Build history of the part. All positions in model axes, mm. A direction names the side the tool comes from. Round coordinates to 2 decimals unless told otherwise and drop trailing zeros. Write each loop counter-clockwise with the first axis right and the second up, starting at its lowest first coordinate (ties: lowest second). Pieces come first, ordered by that corner, then holes.
1) Which spindle directions (+Z, -Z, +X, -X, +Y, -Y) get a long thin tool onto all of the face, cutting with end or side? Do faces 5 (the cylindrical face through (-20.37, -10.4, 2.29)), 6 (the cylindrical face through (4.1, -22.5, 3)), 7 (the cylindrical face through (-14.31, -11.75, 5.7)). Say none if no direction does.
2) Saw through at D-D (x = -9). Write the cut outline in (y, z).
3) Saw through at B-B (z = 2). State how many separate pieces and enclosed holes the cut face has, plus the area to 3 significant figures.
4) Saw through at C-C (x = 0). Write the cut outline in (y, z).
5) Wall check: probe 1 along X at (y, z) = (-2, 3.25); probe 2 along Y at (x, z) = (10.5, 0.5); probe 3 along X at (y, z) = (0, 3.75). Give the ranges that are in metal, low to high.
6) Flat gauge pins, fed straight in: pin 1 (23 mm diameter, centred on x = 0, y = 0, fed in from +Z); pin 2 (2 mm diameter, centred on x = -8.5, z = 4.5, fed in from +Y); pin 3 (3 mm diameter, centred on x = 15.5, y = 10, fed in from +Z); pin 4 (1.5 mm diameter, centred on y = 18, z = 1.5, fed in from +X). Where does each tip first touch, or does it go through?
7) Saw through at A-A (y = 0). Write the cut outline in (x, z).
8) Pull direction Y, two halves, no side cores. Call faces 1 (the flat face through (-14.463, -11.505, 4.458)), 2 (the cylindrical face through (11.42, -22.24, 2.96)), 3 (the flat face through (-16, -8, 4)), 4 (the cylindrical face through (-11.42, 22.24, 2.96)): +Y half, -Y half, draft (parallel to the pull), parting line (faces both ways), or undercut.
from build123d import *

# Parameters (mm, degrees)
SKETCH1_R           = 25
SKETCH1_R_2         = 14.25
BOSS_EXTRUDE1_DEPTH = 6
CUT_EXTRUDE1_REACH  = 8
CUT_EXTRUDE2_REACH  = 8
SKETCH3_R           = 1.5875
CUT_EXTRUDE3_DEPTH  = 2
CUT_EXTRUDE4_START  = -6.000001
SKETCH5_R           = 41.768296762
CUT_EXTRUDE4_DEPTH  = 6.000001
FILLET1_R           = 1


with BuildPart() as part:
    # Sketch1 → Boss-Extrude1 (new body)
    with BuildSketch(Plane.XY):
        Circle(SKETCH1_R)
        Circle(SKETCH1_R_2, mode=Mode.SUBTRACT)
    extrude(amount=BOSS_EXTRUDE1_DEPTH)

    # Sketch2 → Cut-Extrude1 (cut, up to next)
    with BuildSketch(Plane.XY.offset(6), mode=Mode.PRIVATE) as cut_extrude1_sk1:
        with BuildLine():
            Line((-11.636735818, -22.126598914), (9.351350952, -23.185172748))
            ThreePointArc((9.351350952, -23.185172748), (-1.259321499, -24.968262041), (-11.636735818, -22.126598914))
        make_face()
    cut_extrude1_tool1 = extrude(cut_extrude1_sk1.sketch, amount=-CUT_EXTRUDE1_REACH, mode=Mode.PRIVATE) & part.part
    add(cut_extrude1_tool1.solids().sort_by_distance((-1.189534, -23.584609, 6))[0], mode=Mode.SUBTRACT)

    # Sketch3 → Cut-Extrude2 (cut, up to next)
    with BuildSketch(Plane(origin=(0, 0, 0), x_dir=(-1, 0, 0), z_dir=(0, 0, -1)), mode=Mode.PRIVATE) as cut_extrude2_sk1:
        with Locations((11.49485864, -17.913013938)):
            Circle(SKETCH3_R)
    cut_extrude2_tool1 = extrude(cut_extrude2_sk1.sketch, amount=-CUT_EXTRUDE2_REACH, mode=Mode.PRIVATE) & part.part
    add(cut_extrude2_tool1.solids().sort_by_distance((-11.494859, -17.913014, 0))[0], mode=Mode.SUBTRACT)
    # Sketch3 → Cut-Extrude2 (cut, up to next)
    with BuildSketch(Plane(origin=(0, 0, 0), x_dir=(-1, 0, 0), z_dir=(0, 0, -1)), mode=Mode.PRIVATE) as cut_extrude2_sk2:
        with Locations((21.260554449, 0.998332626)):
            Circle(SKETCH3_R)
    cut_extrude2_tool2 = extrude(cut_extrude2_sk2.sketch, amount=-CUT_EXTRUDE2_REACH, mode=Mode.PRIVATE) & part.part
    add(cut_extrude2_tool2.solids().sort_by_distance((-21.260554, 0.998333, 0))[0], mode=Mode.SUBTRACT)
    # Sketch3 → Cut-Extrude2 (cut, up to next)
    with BuildSketch(Plane(origin=(0, 0, 0), x_dir=(-1, 0, 0), z_dir=(0, 0, -1)), mode=Mode.PRIVATE) as cut_extrude2_sk3:
        with Locations((9.765695809, 18.911346564)):
            Circle(SKETCH3_R)
    cut_extrude2_tool3 = extrude(cut_extrude2_sk3.sketch, amount=-CUT_EXTRUDE2_REACH, mode=Mode.PRIVATE) & part.part
    add(cut_extrude2_tool3.solids().sort_by_distance((-9.765696, 18.911347, 0))[0], mode=Mode.SUBTRACT)
    # Sketch3 → Cut-Extrude2 (cut, up to next)
    with BuildSketch(Plane(origin=(0, 0, 0), x_dir=(-1, 0, 0), z_dir=(0, 0, -1)), mode=Mode.PRIVATE) as cut_extrude2_sk4:
        with Locations((-11.49485864, 17.913013938)):
            Circle(SKETCH3_R)
    cut_extrude2_tool4 = extrude(cut_extrude2_sk4.sketch, amount=-CUT_EXTRUDE2_REACH, mode=Mode.PRIVATE) & part.part
    add(cut_extrude2_tool4.solids().sort_by_distance((11.494859, 17.913014, 0))[0], mode=Mode.SUBTRACT)
    # Sketch3 → Cut-Extrude2 (cut, up to next)
    with BuildSketch(Plane(origin=(0, 0, 0), x_dir=(-1, 0, 0), z_dir=(0, 0, -1)), mode=Mode.PRIVATE) as cut_extrude2_sk5:
        with Locations((-21.260554449, -0.998332626)):
            Circle(SKETCH3_R)
    cut_extrude2_tool5 = extrude(cut_extrude2_sk5.sketch, amount=-CUT_EXTRUDE2_REACH, mode=Mode.PRIVATE) & part.part
    add(cut_extrude2_tool5.solids().sort_by_distance((21.260554, -0.998333, 0))[0], mode=Mode.SUBTRACT)
    # Sketch3 → Cut-Extrude2 (cut, up to next)
    with BuildSketch(Plane(origin=(0, 0, 0), x_dir=(-1, 0, 0), z_dir=(0, 0, -1)), mode=Mode.PRIVATE) as cut_extrude2_sk6:
        with Locations((-9.765695809, -18.911346564)):
            Circle(SKETCH3_R)
    cut_extrude2_tool6 = extrude(cut_extrude2_sk6.sketch, amount=-CUT_EXTRUDE2_REACH, mode=Mode.PRIVATE) & part.part
    add(cut_extrude2_tool6.solids().sort_by_distance((9.765696, -18.911347, 0))[0], mode=Mode.SUBTRACT)

    # Sketch4 → Cut-Extrude3 (cut)
    with BuildSketch(Plane.XY.offset(6)):
        Polygon((12.56074277, 10.510839218), (35.025911551, 22.247124987), (38.267200626, 16.04276804), (15.802031846, 4.306482271), (-51.191313487, -30.692277506), (-54.432602563, -24.487920559), align=None)
    extrude(amount=-CUT_EXTRUDE3_DEPTH, mode=Mode.SUBTRACT)

    # Sketch5 → Cut-Extrude4 (cut)
    with BuildSketch(Plane.XY.offset(6).offset(CUT_EXTRUDE4_START)):
        Circle(SKETCH5_R)
        with BuildLine():
            ThreePointArc((-7.9313675, 22.143070177), (-11.470711058, 22.213121974), (-13.462706849, 19.286722677))
            ThreePointArc((-13.462706849, 19.286722677), (-13.698075607, 18.528505361), (-14.209890558, 17.921597291))
            ThreePointArc((-14.209890558, 17.921597291), (-19.249084936, 12.352221187), (-22.212464402, 5.450785662))
            ThreePointArc((-22.212464402, 5.450785662), (-22.550939275, 4.732644513), (-23.142145042, 4.202769347))
            ThreePointArc((-23.142145042, 4.202769347), (-24.972483456, 1.172633811), (-23.434145218, -2.015684796))
            ThreePointArc((-23.434145218, -2.015684796), (-22.89519414, -2.598628778), (-22.62550381, -3.345327563))
            ThreePointArc((-22.62550381, -3.345327563), (-20.32187981, -10.494085961), (-15.826751055, -16.511165622))
            ThreePointArc((-15.826751055, -16.511165622), (-15.374060012, -17.163364035), (-15.210777541, -17.940300831))
            ThreePointArc((-15.210777541, -17.940300831), (-13.501772398, -21.040488163), (-9.97143837, -21.302407473))
            ThreePointArc((-9.97143837, -21.302407473), (-9.197118534, -21.127134139), (-8.415613251, -21.266924854))
            ThreePointArc((-8.415613251, -21.266924854), (-1.072794873, -22.846307148), (6.385713347, -21.961951284))
            ThreePointArc((6.385713347, -21.961951284), (7.176879262, -21.896008547), (7.9313675, -22.143070177))
            ThreePointArc((7.9313675, -22.143070177), (11.470711058, -22.213121974), (13.462706849, -19.286722677))
            ThreePointArc((13.462706849, -19.286722677), (13.698075607, -18.528505361), (14.209890558, -17.921597291))
            ThreePointArc((14.209890558, -17.921597291), (19.249084936, -12.352221187), (22.212464402, -5.450785662))
            ThreePointArc((22.212464402, -5.450785662), (22.550939275, -4.732644513), (23.142145042, -4.202769347))
            ThreePointArc((23.142145042, -4.202769347), (24.972483456, -1.172633811), (23.434145218, 2.015684796))
            ThreePointArc((23.434145218, 2.015684796), (22.89519414, 2.598628778), (22.62550381, 3.345327563))
            ThreePointArc((22.62550381, 3.345327563), (20.100933566, 10.911329384), (15.131770312, 17.150340124))
            ThreePointArc((15.131770312, 17.150340124), (13.824370884, 20.808211783), (9.97143837, 21.302407473))
            ThreePointArc((9.97143837, 21.302407473), (9.197118534, 21.127134139), (8.415613251, 21.266924854))
            ThreePointArc((8.415613251, 21.266924854), (1.072794873, 22.846307148), (-6.385713347, 21.961951284))
            ThreePointArc((-6.385713347, 21.961951284), (-7.176879262, 21.896008547), (-7.9313675, 22.143070177))
        make_face(mode=Mode.SUBTRACT)
    extrude(amount=CUT_EXTRUDE4_DEPTH, mode=Mode.SUBTRACT)

    # Fillet1
    fillet1_edges = [part.edges().sort_by_distance(p)[0] for p in [
        (-14.517589627, -11.533137966, 6),
        (-20.271833071, -10.590440175, 4),
        (14.517589627, 11.533137966, 6),
        (20.271833071, 10.590440175, 4),
        (17.758878703, 5.328781019, 6),
        (-17.758878703, -5.328781019, 6),
    ]]
    fillet(fillet1_edges, radius=FILLET1_R)


solid = part.part
Evaluation:
1. face 5: +Z, -Z, -X, -Y
1. face 6: +Z, -Z, -Y
1. face 7: +Z, -X
2. outline: (-21.13, 0) - (-11.05, 0) - (-11.05, 6) - (-21.13, 6) - close; (11.05, 0) - (17.52, 0) - (17.52, 6) - (11.05, 6) - close; (20.3, 0) - (22.55, 0) - (22.55, 6) - (20.3, 6) - close
3. separate pieces: 1
3. enclosed holes: 7
3. area: 1,020 mm2
4. outline: (-22.71, 0) - (-14.25, 0) - (-14.25, 6) - (-22.71, 6) - close; (14.25, 0) - (22.87, 0) - (22.87, 6) - (14.25, 6) - close
5. probe 1: x = -23.46 to -14.11, 14.11 to 20.03, 22.49 to 24.84
5. probe 2: y = -22.55 to -20.32, -17.5 to -9.63, 9.63 to 16.68, 19.15 to 21.49
5. probe 3: x = -24.84 to -22.49, -20.03 to -14.25, 14.25 to 20.03, 22.49 to 24.84
6. pin 1: passes through
6. pin 2: stops at y = 22.62
6. pin 3: stops at z = 4
6. pin 4: stops at x = 15.21
7. outline: (-24.84, 0) - (-22.49, 0) - (-22.49, 6) - (-24.84, 6) - close; (-20.03, 0) - (-14.25, 0) - (-14.25, 6) - (-20.03, 6) - close; (14.25, 0) - (20.03, 0) - (20.03, 6) - (14.25, 6) - close; (22.49, 0) - (24.84, 0) - (24.84, 6) - (22.49, 6) - close
8. face 1: undercut
8. face 2: -Y half
8. face 3: undercut
8. face 4: +Y half
